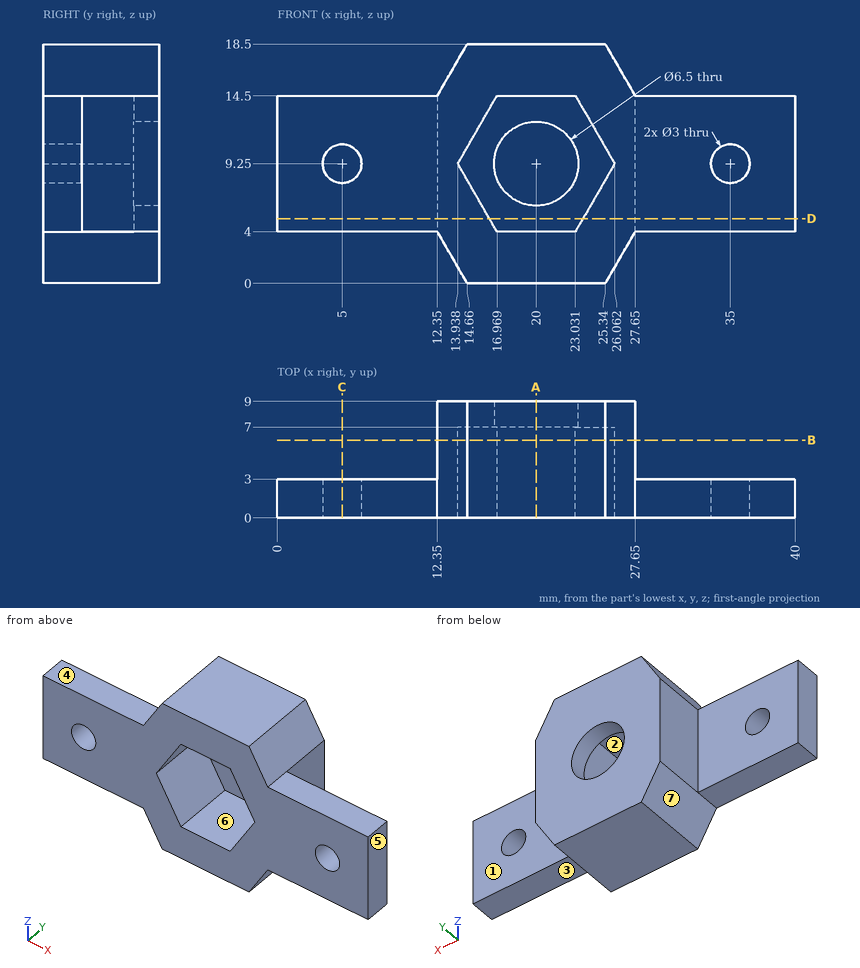
The figure shows three views and two pictorial views of one solid part (mm, origin at its lowest corner). Answer the questions. A direction names the side the tool comes from. Coordinates: 2 decimals unless noted, no trailing zeros. Write each loop counter-clockwise with the first axis right and the second up, starting at its lowest first coordinate (ties: lowest second). Pieces come first, ordered by that corner, then holes.
1. Flat-ended cylindrical pins translate along their axes: pin 1 (5 mm diameter, centred on x = 35, z = 9.25, fed in from +Y); pin 2 (1.5 mm diameter, centred on y = 4, z = 3.5, fed in from +X); pin 3 (4 mm diameter, centred on x = 20, z = 9.25, fed in from +Y); pin 4 (1.5 mm diameter, centred on x = 35.5, y = 2, fed in from -Z). Find the tip coordinate at first contact, or state that the pin passes through.
Results list:
pin 1: stops at y = 3
pin 2: stops at x = 27.65
pin 3: passes through
pin 4: stops at z = 4
2. For a pull along X with two mould halves and no side action, classify the marked faces 5, 6 and 7 as +X half, -X half, draft (parallel to the pull), parting line (faces both ways), or undercut.
Results list:
face 5: +X half
face 6: undercut
face 7: -X half
3. The part is cut by section C-C, the plane x = 5. Write down the section's boundary in (y, z).
Results list:
outline: (0, 4) - (3, 4) - (3, 7.75) - (0, 7.75) - close; (0, 10.75) - (3, 10.75) - (3, 14.5) - (0, 14.5) - close
4. Consider line 1 along X through (y, z) = (0.7, 9.25); line 2 along X through (y, z) = (7.8, 9.25); line 3 along Z through (x, y) = (22.5, 5.5). Determine where each line is inside the solid, lowest interval first.
Results list:
line 1: x = 0 to 3.5, 6.5 to 13.94, 26.06 to 33.5, 36.5 to 40
line 2: x = 12.35 to 16.75, 23.25 to 27.65
line 3: z = 0 to 4, 14.5 to 18.5
5. The part is cut by section A-A, the plane x = 20. Write down the section's boundary in (y, z).
Results list:
outline: (0, 0) - (9, 0) - (9, 6) - (7, 6) - (7, 4) - (0, 4) - close; (0, 14.5) - (7, 14.5) - (7, 12.5) - (9, 12.5) - (9, 18.5) - (0, 18.5) - close
6. The part is cut by section B-B, the plane y = 6. Write down the section's boundary in (x, z).
Results list:
outline: (12.35, 4) - (14.66, 0) - (25.34, 0) - (27.65, 4) - (27.65, 14.5) - (25.34, 18.5) - (14.66, 18.5) - (12.35, 14.5) - close; hole (13.94, 9.25) - (16.97, 4) - (23.03, 4) - (26.06, 9.25) - (23.03, 14.5) - (16.97, 14.5) - close
7. The part is cut by section D-D, the plane z = 5. Write down the section's boundary in (x, y).
Results list:
outline: (0, 0) - (16.39, 0) - (16.39, 7) - (23.61, 7) - (23.61, 0) - (40, 0) - (40, 3) - (27.65, 3) - (27.65, 9) - (12.35, 9) - (12.35, 3) - (0, 3) - close
8. For the marked faces 1, 2, 3 and 4, determine the directions among +Z, -Z, +X, -X, +Y, -Y from which every point of the face is accessible in a straight line to the end or side of a thin tool.
Results list:
face 1: +Z, -Z, +X, +Y
face 2: -Y
face 3: -Z, +X, +Y, -Y
face 4: +Z, -X, +Y, -Y
